Here's how the part is built. I have some questions about the finished solid (model axes, mm). A direction names the side the tool comes from. Round coordinates to 2 decimals unless told otherwise and drop trailing zeros. Answer as CSV lines item,"result".
from build123d import *

# Parameters (mm, degrees)
CYLINDER1694_R     = 17
CYLINDER1694_DEPTH = 160
CYLINDER1713_R     = 4
CYLINDER1713_DEPTH = 100
CYLINDER1712_R     = 4
CYLINDER1712_DEPTH = 100
CYLINDER1696_R     = 1.5
CYLINDER1696_DEPTH = 100
CYLINDER1697_R     = 1.5
CYLINDER1697_DEPTH = 100
CYLINDER1698_R     = 1.5
CYLINDER1698_DEPTH = 100
CYLINDER1699_R     = 1.5
CYLINDER1699_DEPTH = 100
CYLINDER1700_R     = 1.5
CYLINDER1700_DEPTH = 100
CYLINDER1701_R     = 1.5
CYLINDER1701_DEPTH = 100
CYLINDER1702_R     = 1.5
CYLINDER1702_DEPTH = 100
CYLINDER1695_R     = 1.5
CYLINDER1695_DEPTH = 100
CYLINDER1716_R     = 4
CYLINDER1716_DEPTH = 100
CYLINDER1714_R     = 4
CYLINDER1714_DEPTH = 100
CYLINDER1717_R     = 4
CYLINDER1717_DEPTH = 100
CYLINDER1718_R     = 4
CYLINDER1718_DEPTH = 100
CYLINDER1719_R     = 4
CYLINDER1719_DEPTH = 100
CYLINDER1720_R     = 4
CYLINDER1720_DEPTH = 100
CYLINDER1721_R     = 4
CYLINDER1721_DEPTH = 100
CYLINDER1715_R     = 4
CYLINDER1715_DEPTH = 100
CYLINDER1705_R     = 4
CYLINDER1705_DEPTH = 20
CYLINDER1706_R     = 4
CYLINDER1706_DEPTH = 20
CYLINDER1707_R     = 4
CYLINDER1707_DEPTH = 20
CYLINDER1708_R     = 4
CYLINDER1708_DEPTH = 40
CYLINDER1709_R     = 4
CYLINDER1709_DEPTH = 40
CYLINDER1710_R     = 4
CYLINDER1710_DEPTH = 40
CYLINDER1711_R     = 4
CYLINDER1711_DEPTH = 40
CYLINDER1704_R     = 4
CYLINDER1704_DEPTH = 20
CYLINDER1703_R     = 59
CYLINDER1703_DEPTH = 16
CHAMFER059_SIZE    = 4
FILLET003_R        = 4


with BuildPart() as obj1:
    # Cylinder1694 → Cylinder1694 (new body)
    with BuildSketch(Plane(origin=(-18, 0, -60), x_dir=(1, 0, 0), z_dir=(0, 0, 1))):
        Circle(CYLINDER1694_R)
    extrude(amount=CYLINDER1694_DEPTH)


with BuildPart() as obj2:
    # Cylinder1713 → Cylinder1713 (new body)
    with BuildSketch(Plane(origin=(14, 0, -18), x_dir=(1, 0, 0), z_dir=(0, 0, 1))):
        Circle(CYLINDER1713_R)
    extrude(amount=CYLINDER1713_DEPTH)


with BuildPart() as obj3:
    # Cylinder1712 → Cylinder1712 (new body)
    with BuildSketch(Plane(origin=(90, 0, -18), x_dir=(1, 0, 0), z_dir=(0, 0, 1))):
        Circle(CYLINDER1712_R)
    extrude(amount=CYLINDER1712_DEPTH)

    # Compound941: union obj2
    add(obj2.part)


with BuildPart() as obj4:
    # Cylinder1696 → Cylinder1696 (new body)
    with BuildSketch(Plane(origin=(-34, -16, -60), x_dir=(1, 0, 0), z_dir=(0, 0, 1))):
        Circle(CYLINDER1696_R)
    extrude(amount=CYLINDER1696_DEPTH)


with BuildPart() as obj5:
    # Cylinder1697 → Cylinder1697 (new body)
    with BuildSketch(Plane(origin=(34, -16, -60), x_dir=(1, 0, 0), z_dir=(0, 0, 1))):
        Circle(CYLINDER1697_R)
    extrude(amount=CYLINDER1697_DEPTH)


with BuildPart() as obj6:
    # Cylinder1698 → Cylinder1698 (new body)
    with BuildSketch(Plane(origin=(34, 16, -60), x_dir=(1, 0, 0), z_dir=(0, 0, 1))):
        Circle(CYLINDER1698_R)
    extrude(amount=CYLINDER1698_DEPTH)


with BuildPart() as obj7:
    # Cylinder1699 → Cylinder1699 (new body)
    with BuildSketch(Plane(origin=(16, 34, -60), x_dir=(1, 0, 0), z_dir=(0, 0, 1))):
        Circle(CYLINDER1699_R)
    extrude(amount=CYLINDER1699_DEPTH)


with BuildPart() as obj8:
    # Cylinder1700 → Cylinder1700 (new body)
    with BuildSketch(Plane(origin=(10, -36, -60), x_dir=(1, 0, 0), z_dir=(0, 0, 1))):
        Circle(CYLINDER1700_R)
    extrude(amount=CYLINDER1700_DEPTH)


with BuildPart() as obj9:
    # Cylinder1701 → Cylinder1701 (new body)
    with BuildSketch(Plane(origin=(-16, -34, -60), x_dir=(1, 0, 0), z_dir=(0, 0, 1))):
        Circle(CYLINDER1701_R)
    extrude(amount=CYLINDER1701_DEPTH)


with BuildPart() as obj10:
    # Cylinder1702 → Cylinder1702 (new body)
    with BuildSketch(Plane(origin=(-16, 34, -60), x_dir=(1, 0, 0), z_dir=(0, 0, 1))):
        Circle(CYLINDER1702_R)
    extrude(amount=CYLINDER1702_DEPTH)


with BuildPart() as obj11:
    # Cylinder1695 → Cylinder1695 (new body)
    with BuildSketch(Plane(origin=(-34, 16, -60), x_dir=(1, 0, 0), z_dir=(0, 0, 1))):
        Circle(CYLINDER1695_R)
    extrude(amount=CYLINDER1695_DEPTH)

    # Compound938: union obj4, obj5, obj6, obj7, obj8, obj9, obj10
    add(obj4.part)
    add(obj5.part)
    add(obj6.part)
    add(obj7.part)
    add(obj8.part)
    add(obj9.part)
    add(obj10.part)


with BuildPart() as obj12:
    # Cylinder1716 → Cylinder1716 (new body)
    with BuildSketch(Plane(origin=(-16, 34, -90), x_dir=(1, 0, 0), z_dir=(0, 0, 1))):
        Circle(CYLINDER1716_R)
    extrude(amount=CYLINDER1716_DEPTH)


with BuildPart() as obj13:
    # Cylinder1714 → Cylinder1714 (new body)
    with BuildSketch(Plane(origin=(-16, -34, -90), x_dir=(1, 0, 0), z_dir=(0, 0, 1))):
        Circle(CYLINDER1714_R)
    extrude(amount=CYLINDER1714_DEPTH)


with BuildPart() as obj14:
    # Cylinder1717 → Cylinder1717 (new body)
    with BuildSketch(Plane(origin=(34, -16, -90), x_dir=(1, 0, 0), z_dir=(0, 0, 1))):
        Circle(CYLINDER1717_R)
    extrude(amount=CYLINDER1717_DEPTH)


with BuildPart() as obj15:
    # Cylinder1718 → Cylinder1718 (new body)
    with BuildSketch(Plane(origin=(16, 34, -90), x_dir=(1, 0, 0), z_dir=(0, 0, 1))):
        Circle(CYLINDER1718_R)
    extrude(amount=CYLINDER1718_DEPTH)


with BuildPart() as obj16:
    # Cylinder1719 → Cylinder1719 (new body)
    with BuildSketch(Plane(origin=(10, -36, -90), x_dir=(1, 0, 0), z_dir=(0, 0, 1))):
        Circle(CYLINDER1719_R)
    extrude(amount=CYLINDER1719_DEPTH)


with BuildPart() as obj17:
    # Cylinder1720 → Cylinder1720 (new body)
    with BuildSketch(Plane(origin=(-34, 16, -90), x_dir=(1, 0, 0), z_dir=(0, 0, 1))):
        Circle(CYLINDER1720_R)
    extrude(amount=CYLINDER1720_DEPTH)


with BuildPart() as obj18:
    # Cylinder1721 → Cylinder1721 (new body)
    with BuildSketch(Plane(origin=(34, 16, -90), x_dir=(1, 0, 0), z_dir=(0, 0, 1))):
        Circle(CYLINDER1721_R)
    extrude(amount=CYLINDER1721_DEPTH)


with BuildPart() as obj19:
    # Cylinder1715 → Cylinder1715 (new body)
    with BuildSketch(Plane(origin=(-34, -16, -90), x_dir=(1, 0, 0), z_dir=(0, 0, 1))):
        Circle(CYLINDER1715_R)
    extrude(amount=CYLINDER1715_DEPTH)

    # Compound940: union obj12, obj13, obj14, obj15, obj16, obj17, obj18
    add(obj12.part)
    add(obj13.part)
    add(obj14.part)
    add(obj15.part)
    add(obj16.part)
    add(obj17.part)
    add(obj18.part)


with BuildPart() as obj20:
    # Cylinder1705 → Cylinder1705 (new body)
    with BuildSketch(Plane(origin=(103, 12, -20), x_dir=(1, 0, 0), z_dir=(0, 0, 1))):
        Circle(CYLINDER1705_R)
    extrude(amount=CYLINDER1705_DEPTH)


with BuildPart() as obj21:
    # Cylinder1706 → Cylinder1706 (new body)
    with BuildSketch(Plane(origin=(76, 24, -18), x_dir=(1, 0, 0), z_dir=(0, 0, 1))):
        Circle(CYLINDER1706_R)
    extrude(amount=CYLINDER1706_DEPTH)


with BuildPart() as obj22:
    # Cylinder1707 → Cylinder1707 (new body)
    with BuildSketch(Plane(origin=(91, -27, -18), x_dir=(1, 0, 0), z_dir=(0, 0, 1))):
        Circle(CYLINDER1707_R)
    extrude(amount=CYLINDER1707_DEPTH)


with BuildPart() as obj23:
    # Cylinder1708 → Cylinder1708 (new body)
    with BuildSketch(Plane(origin=(13, -27, -18), x_dir=(1, 0, 0), z_dir=(0, 0, 1))):
        Circle(CYLINDER1708_R)
    extrude(amount=CYLINDER1708_DEPTH)


with BuildPart() as obj24:
    # Cylinder1709 → Cylinder1709 (new body)
    with BuildSketch(Plane(origin=(28, 24, -18), x_dir=(1, 0, 0), z_dir=(0, 0, 1))):
        Circle(CYLINDER1709_R)
    extrude(amount=CYLINDER1709_DEPTH)


with BuildPart() as obj25:
    # Cylinder1710 → Cylinder1710 (new body)
    with BuildSketch(Plane(origin=(1, -12, -18), x_dir=(1, 0, 0), z_dir=(0, 0, 1))):
        Circle(CYLINDER1710_R)
    extrude(amount=CYLINDER1710_DEPTH)


with BuildPart() as obj26:
    # Cylinder1711 → Cylinder1711 (new body)
    with BuildSketch(Plane(origin=(1, 12, -18), x_dir=(1, 0, 0), z_dir=(0, 0, 1))):
        Circle(CYLINDER1711_R)
    extrude(amount=CYLINDER1711_DEPTH)


with BuildPart() as obj27:
    # Cylinder1704 → Cylinder1704 (new body)
    with BuildSketch(Plane(origin=(103, -12, -20), x_dir=(1, 0, 0), z_dir=(0, 0, 1))):
        Circle(CYLINDER1704_R)
    extrude(amount=CYLINDER1704_DEPTH)

    # Compound939: union obj20, obj21, obj22, obj23, obj24, obj25, obj26
    add(obj20.part)
    add(obj21.part)
    add(obj22.part)
    add(obj23.part)
    add(obj24.part)
    add(obj25.part)
    add(obj26.part)


with BuildPart() as fillet003:
    # Cylinder1703 → Cylinder1703 (new body)
    with BuildSketch(Plane.XY.offset(2)):
        Circle(CYLINDER1703_R)
    extrude(amount=CYLINDER1703_DEPTH)

    # Cut593: cut obj27
    add(obj27.part, mode=Mode.SUBTRACT)

    # Cut594: cut obj19
    add(obj19.part, mode=Mode.SUBTRACT)

    # Cut595: cut obj11
    add(obj11.part, mode=Mode.SUBTRACT)

    # Chamfer059
    chamfer059_edges = [fillet003.edges().sort_by_distance(p)[0] for p in [
        (-59, 0, 2),
    ]]
    chamfer(chamfer059_edges, length=CHAMFER059_SIZE)

    # Cut596: cut obj3
    add(obj3.part, mode=Mode.SUBTRACT)


with BuildPart() as fillet003_1:
    # Cut596 placement: moved
    add(fillet003.part.moved(Location((0, 0, 4))))

    # Cut585: cut obj1
    add(obj1.part, mode=Mode.SUBTRACT)

    # Fillet003
    fillet003_edges = [fillet003_1.edges().sort_by_distance(p)[0] for p in [
        (-35, 0, 22),
    ]]
    fillet(fillet003_edges, radius=FILLET003_R)


solid = fillet003_1.part
Item 1: I need wall thicknesses on L1, parallel to Y at x = 1, z = 12.75; L2, parallel to X at y = 12.5, z = 8.75; L3, parallel to Y at x = -31, z = 7.5. Which ranges of each line are inside material? Lowest first, please.
Results found:
L1,"y = -58.99 to -16, -8 to 8, 16 to 58.99"
L2,"x = -56.38 to -35.94, -32.06 to -29.52, -6.48 to -2.97, 4.97 to 32.06, 35.94 to 56.38"
L3,"y = -47.24 to -18.65, -13.35 to -10.95, 10.95 to 13.35, 18.65 to 47.24"
Item 2: Will these pins go through, and if not, where does the flat tip stop? pin 1 (6 mm diameter, centred on y = -9, z = 12.5, fed in from -X); pin 2 (1.5 mm diameter, centred on y = 9.5, z = 14.5, fed in from +X); pin 3 (6.5 mm diameter, centred on x = 16, y = 34, fed in from -Z); pin 4 (7 mm diameter, centred on x = 28, y = 24, fed in from +Z).
Results found:
pin 1,"stops at x = -58.69"
pin 2,"stops at x = 58.35"
pin 3,"stops at z = 14"
pin 4,"passes through"
Item 3: For faces 4 (the cylindrical face through (-16.521, 37.966, 9.944)), 5 (the cylindrical face through (32.8, 15.1, 17.9)), which set-ups out of +Z, -Z, +X, -X, +Y, -Y let a thin tool reach every point of the face, with its end or its side?
Results found:
face 4,"-Z"
face 5,"+Z, -Z"
Item 4: If we mould it in two halves opening along X, with no side actions, what happens to faces 1 (the conical face through (52.645, 16.579, 6.194)), 2 (the flat face through (-14, 34, 14)), 3 (the flat face through (12, -12, 22))? For each: pulls with the +X half, pulls with the -X half, needs draft (parallel to the pull), parting line crosses it, or undercut.
Results found:
face 1,"parting line crosses it"
face 2,"undercut"
face 3,"needs draft"
Item 5: Suppose I cut it at A-A, the plane z = 15.75. State how many separate pieces and enclosed holes the cut face has, then the cut area to 3 significant figures.
Results found:
separate pieces,"1"
enclosed holes,"14"
area,"9,720 mm²"
